Check sheet for the modelled part. Datum: model origin and axes. Units: mm. A direction names the side the tool comes from. Give positions to 0.01 mm unless a question says otherwise; leave off trailing zeros. Order: outer loops, then holes, each group sorted by start corner. A loop starts at its lowest first (then second) coordinate and runs counter-clockwise, first axis right, second up. Notation, with made-up numbers: (30.5, 39.25) -> (41.5, 39.25) arc R17 cw to (41.5, 53.25) -> close; hole circle Ø8 at (35, -17). An arc over 180 degrees is marked (long way). One line per question, with ' | ' between items.
```python
from build123d import *

# Parameters (mm, degrees)
CYLINDER_R        = 7.25
CYLINDER_DEPTH    = 49.8
CYLINDER003_R     = 1.5
CYLINDER003_DEPTH = 1
CYLINDER001_R     = 5.25
CYLINDER001_DEPTH = 45.8
CYLINDER002_R     = 5
CYLINDER002_DEPTH = 45.8
BOX_W             = 9
BOX_H             = 0.01
BOX_DEPTH         = 2
BOX006_W          = 9
BOX006_H          = 3
BOX006_DEPTH      = 8
BOX002_W          = 15
BOX002_H          = 10
BOX002_DEPTH      = 49.8
BOX003_W          = 10.5
BOX003_H          = 1.5
BOX003_DEPTH      = 49.8
CHAMFER_SIZE      = 1.499
FILLET_R          = 3.75
BOX004_W          = 2.75
BOX004_H          = 0.1
BOX004_DEPTH      = 5
BOX005_W          = 2.75
BOX005_H          = 0.1
BOX005_DEPTH      = 5
CYLINDER004_R     = 1
CYLINDER004_DEPTH = 4
CYLINDER005_R     = 1.5
CYLINDER005_DEPTH = 2
CYLINDER006_R     = 1.5
CYLINDER006_DEPTH = 2


with BuildPart() as part:
    # Cylinder → Cylinder (join)
    with BuildSketch(Plane.XY):
        Circle(CYLINDER_R)
    extrude(amount=CYLINDER_DEPTH)

    # Cylinder003 → Cylinder003 (join)
    with BuildSketch(Plane.XY.offset(-0.8)):
        Circle(CYLINDER003_R)
    extrude(amount=CYLINDER003_DEPTH)

    # Cylinder001 → Cylinder001 (cut)
    with BuildSketch(Plane.XY.offset(2)):
        Circle(CYLINDER001_R)
    extrude(amount=CYLINDER001_DEPTH, mode=Mode.SUBTRACT)

    # Cylinder002 → Cylinder002 (cut)
    with BuildSketch(Plane(origin=(0, 5, 2), x_dir=(1, 0, 0), z_dir=(0, 0, 1))):
        Circle(CYLINDER002_R)
    extrude(amount=CYLINDER002_DEPTH, mode=Mode.SUBTRACT)

    # Box → Box (cut)
    with BuildSketch(Plane(origin=(-4.5, -5, 0), x_dir=(1, 0, 0), z_dir=(0, 0, 1))):
        with Locations((4.5, 0.005)):
            Rectangle(BOX_W, BOX_H)
    extrude(amount=BOX_DEPTH, mode=Mode.SUBTRACT)

    # Box006 → Box006 (cut)
    with BuildSketch(Plane(origin=(-4.5, -2, 2), x_dir=(1, 0, 0), z_dir=(0, 0, 1))):
        with Locations((4.5, 1.5)):
            Rectangle(BOX006_W, BOX006_H)
    extrude(amount=BOX006_DEPTH, mode=Mode.SUBTRACT)

    # Box002 → Box002 (cut)
    with BuildSketch(Plane(origin=(-7.5, -15, 0), x_dir=(1, 0, 0), z_dir=(0, 0, 1))):
        with Locations((7.5, 5)):
            Rectangle(BOX002_W, BOX002_H)
    extrude(amount=BOX002_DEPTH, mode=Mode.SUBTRACT)

    # Box003 → Box003 (join)
    with BuildSketch(Plane(origin=(-5.25, -6.5, 0), x_dir=(1, 0, 0), z_dir=(0, 0, 1))):
        with Locations((5.25, 0.75)):
            Rectangle(BOX003_W, BOX003_H)
    extrude(amount=BOX003_DEPTH)

    # Chamfer
    chamfer_edges = [part.edges().sort_by_distance(p)[0] for p in [
        (5.25, -6.5, 24.9),
        (-5.25, -6.5, 24.9),
    ]]
    chamfer(chamfer_edges, length=CHAMFER_SIZE)

    # Fillet
    fillet_edges = [part.edges().sort_by_distance(p)[0] for p in [
        (3.751, -6.5, 24.9),
        (-3.751, -6.5, 24.9),
    ]]
    fillet(fillet_edges, radius=FILLET_R)

    # Box004 → Box004 (join)
    with BuildSketch(Plane(origin=(-5, -5, 10), x_dir=(1, 0, 0), z_dir=(0, 0, 1))):
        with Locations((1.375, 0.05)):
            Rectangle(BOX004_W, BOX004_H)
    extrude(amount=BOX004_DEPTH)

    # Box005 → Box005 (join)
    with BuildSketch(Plane(origin=(2.25, -5, 10), x_dir=(1, 0, 0), z_dir=(0, 0, 1))):
        with Locations((1.375, 0.05)):
            Rectangle(BOX005_W, BOX005_H)
    extrude(amount=BOX005_DEPTH)

    # Cylinder004 → Cylinder004 (cut)
    with BuildSketch(Plane(origin=(0, 2, -1.55), x_dir=(1, 0, 0), z_dir=(0, -1, 0))):
        Circle(CYLINDER004_R)
    extrude(amount=CYLINDER004_DEPTH, mode=Mode.SUBTRACT)

    # Cylinder005 → Cylinder005 (cut)
    with BuildSketch(Plane(origin=(0, -3.2, 0), x_dir=(1, 0, 0), z_dir=(0, 0, 1))):
        Circle(CYLINDER005_R)
    extrude(amount=CYLINDER005_DEPTH, mode=Mode.SUBTRACT)

    # Cylinder006 → Cylinder006 (cut)
    with BuildSketch(Plane(origin=(0, 3.2, 0), x_dir=(1, 0, 0), z_dir=(0, 0, 1))):
        Circle(CYLINDER006_R)
    extrude(amount=CYLINDER006_DEPTH, mode=Mode.SUBTRACT)


solid = part.part
```
Q1. Thickness scan on line 1 (Z direction, x = 1, y = 2); line 2 (X direction, y = 4.75, z = 2.5); line 3 (X direction, y = 4.25, z = 14). Record the ranges inside material, lowest first.
Result sheet:
line 1: z = 0 to 2, 47.8 to 49.8 | line 2: x = -5.48 to -4.99, 4.99 to 5.48 | line 3: x = -5.87 to -4.94, 4.94 to 5.87
Q2. Depth check by flat-ended pin: pin 1 Ø6 at (x, y) = (6, -1) entering from -Z; pin 2 Ø2.5 at (x, z) = (-1, 19) entering from +Y; pin 3 Ø4 at (y, z) = (-3, 18) entering from -X. Enter the tip coordinate at first touch or a pass-through.
Result sheet:
pin 1: stops at z = 0 | pin 2: stops at y = -4.74 | pin 3: stops at x = -7.18
Q3. Section check B-B (y = -4). Enter the section's corners in (x, z), and give its area (3 significant figures).
Result sheet:
outline: (-6.05, 0) -> (-1.27, 0) -> (-1.27, 2) -> (-3.4, 2) -> (-3.4, 47.8) -> (3.4, 47.8) -> (3.4, 2) -> (1.27, 2) -> (1.27, 0) -> (6.05, 0) -> (6.05, 49.8) -> (-6.05, 49.8) -> close | area: 286 mm2
Q4. Access from +Z, -Z, +X, -X, +Y, -Y to the whole of each face (thin tool, end or side, straight path). Record for faces 4 (the face through (4.9, -1.88, 24.58)), 5 (the face through (-1, 0, -0.8)), 6 (the face through (0.69, -1.33, -0.41)).
Result sheet:
face 4: none | face 5: -Z, +X, -X, +Y, -Y | face 6: -Z
Q5. Mould release check, pull along X, two halves, no side actions. Record for faces 1 (the face through (1, 0, -0.8)), 2 (the face through (-1.11, -2.19, 0.99)), 3 (the face through (-3.652, -6.207, 25.249)): pulls with the +X half, pulls with the -X half, needs draft (parallel to the pull), parting line crosses it, or undercut.
Result sheet:
face 1: needs draft | face 2: undercut | face 3: pulls with the -X half
Q6. Section check A-A (x = 0). Enter the section's corners in (y, z).
Result sheet:
outline: (-6.5, 0) -> (-5, 0) -> (-5, 47.8) -> (7.25, 47.8) -> (7.25, 49.8) -> (-6.5, 49.8) -> close; (-4.99, 0) -> (-4.7, 0) -> (-4.7, 2) -> (-4.99, 2) -> close; (-1.7, 0) -> (-1.5, 0) -> (-1.5, -0.55) -> (1.5, -0.55) -> (1.5, 0) -> (1.7, 0) -> (1.7, 2) -> (-1.7, 2) -> close; (4.7, 0) -> (7.25, 0) -> (7.25, 2) -> (4.7, 2) -> close
